For this review, take the finished solid that the model builds, in its own axes (mm). Round coordinates to 2 decimals unless told otherwise and drop trailing zeros. Loops run counter-clockwise (first coordinate to the right, second up) from the corner with the lowest first, then second, coordinate; pieces in that order, holes last.
1) Take a section at A-A (x = -100). State the section outline as (y, z) points, then the cut area to 3 significant figures.
2) Take a section at B-B (y = -10). State the section outline as (x, z) points.
3) Wall thickness on L1, parallel to Y at x = -100, z = 0.75; L2, parallel to Y at x = -100.5, z = 0.3; L3, parallel to X at y = -4, z = 0.9: over which ranges is each line inside the solid? List them lowest first.
4) Take a section at C-C (x = -110). State the section outline as (y, z) points.
5) Take a section at D-D (z = 0.55). Give the number of separate pieces and of enclosed holes in the cut face, then the cut area to 3 significant figures.
6) Insertion check: pin 1 (0.6 mm diameter, centred on x = -84, z = 1.5, fed in from +Y); pin 2 (0.6 mm diameter, centred on x = -116.5, z = 1, fed in from +Y); pin 3 (1 mm diameter, centred on x = -105, z = 1, fed in from -Y). Each pin has a flat end and moves straight along its axis. Give the tip position at first contact, or say it passes through.
```python
from build123d import *

# Parameters (mm, degrees)
SKETCH1_W           = 3.1
SKETCH1_H           = 1.7
BOSS_EXTRUDE1_DEPTH = 2
CUT_EXTRUDE1_REACH  = 122.95
SKETCH2_R           = 4.5
BOSS_EXTRUDE2_DEPTH = 2
CUT_EXTRUDE2_REACH  = 124.935
SKETCH3_R           = 1.6


with BuildPart() as part:
    # Sketch1 → Boss-Extrude1 (new body)
    with BuildSketch(Plane.XY):
        with BuildLine():
            Line((-105.199970129, 14.069836909), (-120, 8.6))
            Line((-120, 8.6), (-120, -8.6))
            Line((-120, -8.6), (-105.199970129, -14.069836909))
            ThreePointArc((-105.199970129, -14.069836909), (-100, -15), (-94.800029871, -14.069836909))
            Line((-94.800029871, -14.069836909), (-80, -8.6))
            Line((-80, -8.6), (-80, 8.6))
            Line((-80, 8.6), (-94.800029871, 14.069836909))
            ThreePointArc((-94.800029871, 14.069836909), (-100, 15), (-105.199970129, 14.069836909))
        make_face()
        with Locations((-116.5, 5.8)):
            Rectangle(SKETCH1_W, SKETCH1_H, mode=Mode.SUBTRACT)
        with Locations((-83.5, 5.8)):
            Rectangle(SKETCH1_W, SKETCH1_H, mode=Mode.SUBTRACT)
        with Locations((-116.5, -5.8)):
            Rectangle(SKETCH1_W, SKETCH1_H, mode=Mode.SUBTRACT)
        with Locations((-83.5, -5.8)):
            Rectangle(SKETCH1_W, SKETCH1_H, mode=Mode.SUBTRACT)
    extrude(amount=BOSS_EXTRUDE1_DEPTH)

    # Sketch2 → Cut-Extrude1 (cut, up to next)
    with BuildSketch(Plane.XY.offset(2), mode=Mode.PRIVATE) as cut_extrude1_sk1:
        with Locations((-100, 0)):
            Circle(SKETCH2_R)
    cut_extrude1_tool1 = extrude(cut_extrude1_sk1.sketch, amount=-CUT_EXTRUDE1_REACH, mode=Mode.PRIVATE) & part.part
    # Sketch2 → Cut-Extrude1 (cut, up to next)
    with BuildSketch(Plane.XY.offset(2), mode=Mode.PRIVATE) as cut_extrude1_sk2:
        with BuildLine():
            Line((-108, -1.6), (-109.5, -1.6))
            ThreePointArc((-109.5, -1.6), (-111.1, 0), (-109.5, 1.6))
            Line((-109.5, 1.6), (-108, 1.6))
            ThreePointArc((-108, 1.6), (-106.4, 0), (-108, -1.6))
        make_face()
    cut_extrude1_tool2 = extrude(cut_extrude1_sk2.sketch, amount=-CUT_EXTRUDE1_REACH, mode=Mode.PRIVATE) & part.part
    # Sketch2 → Cut-Extrude1 (cut, up to next)
    with BuildSketch(Plane.XY.offset(2), mode=Mode.PRIVATE) as cut_extrude1_sk3:
        with BuildLine():
            Line((-101.6, 8), (-101.6, 9.5))
            ThreePointArc((-101.6, 9.5), (-100, 11.1), (-98.4, 9.5))
            Line((-98.4, 9.5), (-98.4, 8))
            ThreePointArc((-98.4, 8), (-100, 6.4), (-101.6, 8))
        make_face()
    cut_extrude1_tool3 = extrude(cut_extrude1_sk3.sketch, amount=-CUT_EXTRUDE1_REACH, mode=Mode.PRIVATE) & part.part
    # Sketch2 → Cut-Extrude1 (cut, up to next)
    with BuildSketch(Plane.XY.offset(2), mode=Mode.PRIVATE) as cut_extrude1_sk4:
        with BuildLine():
            Line((-92, 1.6), (-90.5, 1.6))
            ThreePointArc((-90.5, 1.6), (-88.9, 0), (-90.5, -1.6))
            Line((-90.5, -1.6), (-92, -1.6))
            ThreePointArc((-92, -1.6), (-93.6, 0), (-92, 1.6))
        make_face()
    cut_extrude1_tool4 = extrude(cut_extrude1_sk4.sketch, amount=-CUT_EXTRUDE1_REACH, mode=Mode.PRIVATE) & part.part
    # Sketch2 → Cut-Extrude1 (cut, up to next)
    with BuildSketch(Plane.XY.offset(2), mode=Mode.PRIVATE) as cut_extrude1_sk5:
        with BuildLine():
            Line((-98.4, -8), (-98.4, -9.5))
            ThreePointArc((-98.4, -9.5), (-100, -11.1), (-101.6, -9.5))
            Line((-101.6, -9.5), (-101.6, -8))
            ThreePointArc((-101.6, -8), (-100, -6.4), (-98.4, -8))
        make_face()
    cut_extrude1_tool5 = extrude(cut_extrude1_sk5.sketch, amount=-CUT_EXTRUDE1_REACH, mode=Mode.PRIVATE) & part.part
    add(cut_extrude1_tool1.solids().sort_by_distance((-100, 0, 2))[0], mode=Mode.SUBTRACT)
    add(cut_extrude1_tool2.solids().sort_by_distance((-108.75, 0, 2))[0], mode=Mode.SUBTRACT)
    add(cut_extrude1_tool3.solids().sort_by_distance((-100, 8.75, 2))[0], mode=Mode.SUBTRACT)
    add(cut_extrude1_tool4.solids().sort_by_distance((-91.25, 0, 2))[0], mode=Mode.SUBTRACT)
    add(cut_extrude1_tool5.solids().sort_by_distance((-100, -8.75, 2))[0], mode=Mode.SUBTRACT)

    # Sketch5 → Boss-Extrude2 (add)
    with BuildSketch(Plane.XY.offset(2)):
        with BuildLine():
            Line((-120, 8.6), (-120, -8.6))
            ThreePointArc((-120, -8.6), (-122, 0), (-120, 8.6))
        make_face()
        with BuildLine():
            Line((-80, 8.6), (-80, -8.6))
            ThreePointArc((-80, -8.6), (-78, 0), (-80, 8.6))
        make_face()
    extrude(amount=-BOSS_EXTRUDE2_DEPTH)

    # Sketch3 → Cut-Extrude2 (cut, up to next)
    with BuildSketch(Plane.XY.offset(2), mode=Mode.PRIVATE) as cut_extrude2_sk1:
        with Locations((-118.05, 0)):
            Circle(SKETCH3_R)
    cut_extrude2_tool1 = extrude(cut_extrude2_sk1.sketch, amount=-CUT_EXTRUDE2_REACH, mode=Mode.PRIVATE) & part.part
    # Sketch3 → Cut-Extrude2 (cut, up to next)
    with BuildSketch(Plane.XY.offset(2), mode=Mode.PRIVATE) as cut_extrude2_sk2:
        with Locations((-81.95, 0)):
            Circle(SKETCH3_R)
    cut_extrude2_tool2 = extrude(cut_extrude2_sk2.sketch, amount=-CUT_EXTRUDE2_REACH, mode=Mode.PRIVATE) & part.part
    add(cut_extrude2_tool1.solids().sort_by_distance((-118.05, 0, 2))[0], mode=Mode.SUBTRACT)
    add(cut_extrude2_tool2.solids().sort_by_distance((-81.95, 0, 2))[0], mode=Mode.SUBTRACT)


solid = part.part
```
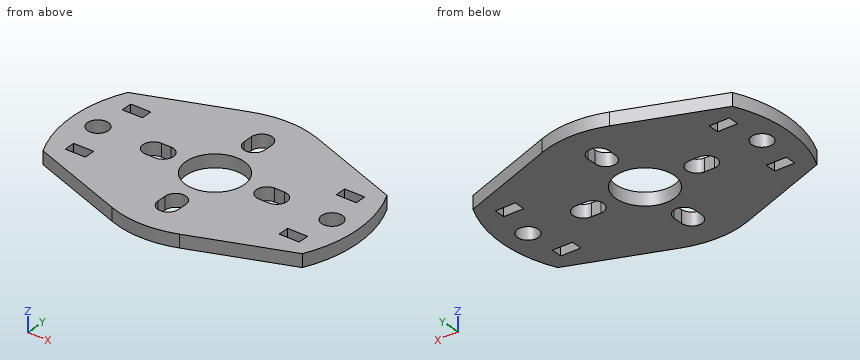
Response:
1. outline: (-15, 0) - (-11.1, 0) - (-11.1, 2) - (-15, 2) - close; (-6.4, 0) - (-4.5, 0) - (-4.5, 2) - (-6.4, 2) - close; (4.5, 0) - (6.4, 0) - (6.4, 2) - (4.5, 2) - close; (11.1, 0) - (15, 0) - (15, 2) - (11.1, 2) - close
1. area: 23.2 mm2
2. outline: (-116.21, 0) - (-101.52, 0) - (-101.52, 2) - (-116.21, 2) - close; (-98.48, 0) - (-83.79, 0) - (-83.79, 2) - (-98.48, 2) - close
3. L1: y = -15 to -11.1, -6.4 to -4.5, 4.5 to 6.4, 11.1 to 15
3. L2: y = -14.99 to -11.02, -6.48 to -4.47, 4.47 to 6.48, 11.02 to 14.99
3. L3: x = -121.59 to -102.06, -97.94 to -78.41
4. outline: (-12.3, 0) - (-1.52, 0) - (-1.52, 2) - (-12.3, 2) - close; (1.52, 0) - (12.3, 0) - (12.3, 2) - (1.52, 2) - close
5. separate pieces: 1
5. enclosed holes: 11
5. area: 871 mm2
6. pin 1: stops at y = 10.19
6. pin 2: stops at y = 10
6. pin 3: stops at y = -14.31
